For this review, take the finished solid that the model builds, in its own axes (mm). A direction names the side the tool comes from. Give positions to 0.01 mm unless a question says otherwise; leave off trailing zeros. Order: outer loops, then holes, each group sorted by start corner. A loop starts at its lowest first (then second) coordinate and runs counter-clockwise, first axis right, second up.
Item 1: Consider section C-C (y = -16). Give the boundary of the cut face in (x, z), plus the area to 3 significant figures.
Item 2: The part is to be moulded in two halves that separate along X. For faces 3 (the cylindrical face through (-4.25, -16.9, 25.3)), 4 (the cylindrical face through (0.81, -16.95, 19.55)), 5 (the flat face through (0, -17, 26.35)), 6 (the flat face through (5.25, -5.6, 3.8)), say which applies: released by +X, released by -X, zero draft, split by the parting line, or undercut.
Item 3: Machinability: for faces 1 (the flat face through (0, 4, 4)), 2 (the flat face through (0, 18.925, 2)), which of the approach directions +Z, -Z, +X, -X, +Y, -Y give a long, thin tool a straight path to every point of the face, cutting with its end or side? Answer none if there is none.
Item 4: Consider section B-B (x = 0). Give the boundary of the cut face in (y, z) (3 decimals).
Item 5: Consider section D-D (x = 4). Give the boundary of the cut face in (y, z) (3 decimals), plus the area to 3 significant figures.
Item 6: For probe 1 along Z at (x, y) = (-3.5, -6); probe 2 along Y at (x, z) = (2.5, 11.5) (3 decimals); probe 3 along Y at (x, z) = (0, 2.55) (3 decimals), list the stretches that pass through material, from the lowest coordinate up.
Item 7: Consider section A-A (z = 21.1). Give the boundary of the cut face in (x, y) (3 decimals), plus the area to 3 significant figures.
Item 8: For P1, Ø5.5, axis at x = 0, z = 21.1, coming from the +Y side (3 decimals), flat-tipped, find the tip position at first contact; note if it passes through.
```python
from build123d import *

# Parameters (mm, degrees)
ESQUISSE1_W             = 10.5
ESQUISSE1_H             = 37.85
ESQUISSE1_R             = 1.75
BOSS_EXTRU_1_DEPTH      = 4
ESQUISSE2_W             = 10.5
ESQUISSE2_H             = 4
BOSS_EXTRU_2_DEPTH      = 22.35
ENL_V_MAT_EXTRU_1_REACH = 39.85
ESQUISSE3_R             = 1.75
CONG_1_R                = 3.5
CONG_2_R                = 4
CONG_3_R                = 8


with BuildPart() as part:
    # Esquisse1 → Boss.-Extru.1 (new body)
    with BuildSketch(Plane.XY):
        Rectangle(ESQUISSE1_W, ESQUISSE1_H)
        with Locations((0, 13.675)):
            Circle(ESQUISSE1_R, mode=Mode.SUBTRACT)
    extrude(amount=BOSS_EXTRU_1_DEPTH)

    # Esquisse2 → Boss.-Extru.2 (add)
    with BuildSketch(Plane.XY.offset(4)):
        with Locations((0, -16.925)):
            Rectangle(ESQUISSE2_W, ESQUISSE2_H)
    extrude(amount=BOSS_EXTRU_2_DEPTH)

    # Esquisse3 → Enlèv. mat.-Extru.1 (cut, up to next)
    with BuildSketch(Plane.XZ.offset(18.925), mode=Mode.PRIVATE) as enl_v_mat_extru_1_sk1:
        with Locations((0, 21.1)):
            Circle(ESQUISSE3_R)
    enl_v_mat_extru_1_tool1 = extrude(enl_v_mat_extru_1_sk1.sketch, amount=-ENL_V_MAT_EXTRU_1_REACH, mode=Mode.PRIVATE) & part.part
    add(enl_v_mat_extru_1_tool1.solids().sort_by_distance((0, -18.925, 21.1))[0], mode=Mode.SUBTRACT)

    # Congé1
    cong_1_edges = [part.edges().sort_by_distance(p)[0] for p in [
        (-5.25, -16.925, 26.35),
        (5.25, -16.925, 26.35),
        (-5.25, 18.925, 2),
        (5.25, 18.925, 2),
    ]]
    fillet(cong_1_edges, radius=CONG_1_R)

    # Congé2
    cong_2_edges = [part.edges().sort_by_distance(p)[0] for p in [
        (0, -14.925, 4),
    ]]
    fillet(cong_2_edges, radius=CONG_2_R)

    # Congé3
    cong_3_edges = [part.edges().sort_by_distance(p)[0] for p in [
        (0, -18.925, 0),
    ]]
    fillet(cong_3_edges, radius=CONG_3_R)


solid = part.part
```
Resolved:
1. outline: (-5.25, 1.82) - (5.25, 1.82) - (5.25, 22.85) arc R3.5 ccw to (1.75, 26.35) - (-1.75, 26.35) arc R3.5 ccw to (-5.25, 22.85) - close; hole circle Ø3.5 at (0, 21.1)
1. area: 243 mm2
2. face 3: released by -X
2. face 4: undercut
2. face 5: zero draft
2. face 6: released by +X
3. face 1: +Z, +X, -X, +Y
3. face 2: +Z, -Z, +X, -X, +Y
4. outline: (-18.925, 8) arc R8 ccw to (-10.925, 0) - (11.925, 0) - (11.925, 4) - (-10.925, 4) arc R4 cw to (-14.925, 8) - (-14.925, 19.35) - (-18.925, 19.35) - close; (-18.925, 22.85) - (-14.925, 22.85) - (-14.925, 26.35) - (-18.925, 26.35) - close; (15.425, 0) - (18.925, 0) - (18.925, 4) - (15.425, 4) - close
5. outline: (-18.925, 8) arc R8 ccw to (-10.925, 0) - (18.106, 0) - (18.106, 4) - (-10.925, 4) arc R4 cw to (-14.925, 8) - (-14.925, 25.531) - (-18.925, 25.531) - close
5. area: 224 mm2
6. probe 1: z = 0 to 4
6. probe 2: y = -18.925 to -14.925
6. probe 3: y = -16.781 to 11.925, 15.425 to 18.925
7. outline: (-5.25, -18.925) - (-1.75, -18.925) - (-1.75, -14.925) - (-5.25, -14.925) - close; (1.75, -18.925) - (5.25, -18.925) - (5.25, -14.925) - (1.75, -14.925) - close
7. area: 28.0 mm2
8. P1: stops at y = -14.925
